CAD build for the part. Positions are in the model's coordinates, mm. Face numbers are marked on the shaded views. A direction names the side the tool comes from. Give positions to 0.01 mm unless a question says otherwise; leave off trailing zeros. Order: outer loops, then holes, each group sorted by start corner. A loop starts at its lowest first (then second) coordinate and runs counter-clockwise, first axis right, second up. Notation, with made-up numbers: (89, 50) -> (136, 50) arc R23 cw to (136, 78) -> close; hole circle Ø9 at (-4.5, 73). An arc over 180 degrees is marked (long way). Use one line per item in the form item = value. Start each with the question number.
1) Tool access for the marked faces 4 and 5: list every direction of +Z, -Z, +X, -X, +Y, -Y with a clear straight run to the whole face (end or side of a thin tool).
2) Cut at A-A, the plane y = 0. Give the cut face in (x, z), and give its area (3 significant figures).
3) Probe line 1 (Z direction, x = 22, y = 0); line 2 (Z direction, x = 4, y = -0.45); line 3 (X direction, y = 0, z = 0.85). List the from-to ranges inside material, lowest first.
4) Drop flat-ended pins along their axis: P1, Ø0.6, axis at x = -1.5, z = -2, coming from the -Y side; P2, Ø0.9, axis at x = -1, z = 2, coming from the -Y side; P3, Ø0.6, axis at x = -1.5, z = -2, coming from the +Y side. Give the stop position or say it passes through.
5) Cut at C-C, the plane x = 23. Give the cut face in (y, z), and give its area (3 significant figures).
6) Mould opens along X. For the marked faces 1, 2 and 3 say: pulls with the +X half, pulls with the -X half, needs draft (parallel to the pull), parting line crosses it, or undercut.
7) Cut at B-B, the plane x = 13.5. Give the cut face in (y, z).
from build123d import *

# Parameters (mm, degrees)
CUT_EXTRUDE1_DEPTH = 2.16
SKETCH3_W          = 4.8
SKETCH3_H          = 0.88
CUT_EXTRUDE2_DEPTH = 2.16


with BuildPart() as part:
    # Sketch1 → Revolve1 (revolve)
    with BuildSketch(Plane.XY):
        with BuildLine():
            Line((-1.591709623, 0), (-2.4, 1.4))
            ThreePointArc((-2.4, 1.4), (-2.158282604, 2.05476512), (-1.827743487, 2.669491525))
            ThreePointArc((-1.827743487, 2.669491525), (-1.726160805, 2.765211773), (-1.590989852, 2.8))
            Line((-1.590989852, 2.8), (0, 2.8))
            Line((0, 2.8), (0, 1.3))
            Line((0, 1.3), (18.1065, 1.3))
            Line((18.1065, 1.3), (18.3065, 1.5))
            Line((18.3065, 1.5), (24.6935, 1.5))
            Line((24.6935, 1.5), (25, 1.1935))
            Line((25, 1.1935), (25, 0))
            Line((25, 0), (-1.591709623, 0))
        make_face()
    revolve(axis=Axis((25, 0, 0), (-1, 0, 0)))

    # Sketch2 → Cut-Extrude1 (cut)
    with BuildSketch(Plane(origin=(-2.4, 0, 0), x_dir=(0, 0, -1), z_dir=(1, 0, 0))):
        with BuildLine():
            ThreePointArc((-1.162126056, -0.356363636), (-1.212435563, -0.700000003), (-0.889682983, -0.828248867))
            ThreePointArc((-0.889682983, -0.828248867), (-0.504218428, -0.873331943), (-0.272443066, -1.184612505))
            ThreePointArc((-0.272443066, -1.184612505), (-6e-09, -1.4), (0.272443063, -1.184612516))
            ThreePointArc((0.272443063, -1.184612516), (0.504218427, -0.873331944), (0.88968299, -0.828248869))
            ThreePointArc((0.88968299, -0.828248869), (1.212435563, -0.700000005), (1.162126064, -0.356363644))
            ThreePointArc((1.162126064, -0.356363644), (1.008436863, -6e-09), (1.162126056, 0.356363636))
            ThreePointArc((1.162126056, 0.356363636), (1.212435565, 0.7), (0.88968299, 0.828248869))
            ThreePointArc((0.88968299, 0.828248869), (0.504218435, 0.873331939), (0.272443068, 1.184612496))
            ThreePointArc((0.272443068, 1.184612496), (7e-09, 1.4), (-0.272443065, 1.18461251))
            ThreePointArc((-0.272443065, 1.18461251), (-0.504218432, 0.873331941), (-0.889682997, 0.828248871))
            ThreePointArc((-0.889682997, 0.828248871), (-1.212435569, 0.699999994), (-1.162126051, 0.356363631))
            ThreePointArc((-1.162126051, 0.356363631), (-1.008436863, -4e-09), (-1.162126056, -0.356363636))
        make_face()
    extrude(amount=CUT_EXTRUDE1_DEPTH, mode=Mode.SUBTRACT)

    # Sketch3 → Cut-Extrude2 (cut)
    with BuildSketch(Plane(origin=(-2.4, 0, 0), x_dir=(0, 0, -1), z_dir=(1, 0, 0))):
        Rectangle(SKETCH3_W, SKETCH3_H)
    extrude(amount=CUT_EXTRUDE2_DEPTH, mode=Mode.SUBTRACT)


solid = part.part
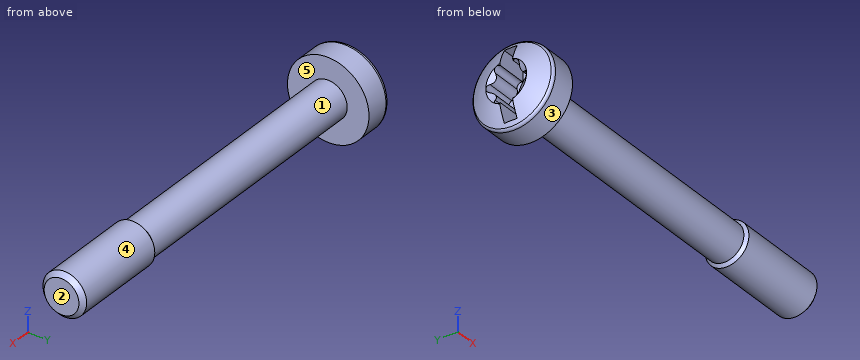
Result:
q1.face_4 = +X
q1.face_5 = none
q2.outline = (-1.99, -2.4) arc R5 ccw to (-1.83, -2.67) arc R0.28 ccw to (-1.59, -2.8) -> (0, -2.8) -> (0, -1.3) -> (18.11, -1.3) -> (18.31, -1.5) -> (24.69, -1.5) -> (25, -1.19) -> (25, 1.19) -> (24.69, 1.5) -> (18.31, 1.5) -> (18.11, 1.3) -> (0, 1.3) -> (0, 2.8) -> (-1.59, 2.8) arc R0.28 ccw to (-1.83, 2.67) arc R5 ccw to (-1.99, 2.4) -> (-0.24, 2.4) -> (-0.24, -2.4) -> close
q2.area = 70.3 mm²
q3.line_1 = -1.5 to 1.5
q3.line_2 = -1.22 to 1.22
q3.line_3 = -0.24 to 25
q4.P1 = -2.22
q4.P2 = -2.33
q4.P3 = 2.22
q5.outline = circle Ø3 at (0, 0)
q5.area = 7.07 mm²
q6.face_1 = undercut
q6.face_2 = pulls with the +X half
q6.face_3 = needs draft
q7.outline = circle Ø2.6 at (0, 0)
